Can you work these out from the model? Positions are in its coordinate system, mm. Coordinates: 2 decimals unless noted, no trailing zeros. Write each loop counter-clockwise with the first axis right and the second up, starting at its lowest first coordinate (ties: lowest second). Pieces come first, ordered by that corner, then holes.
```python
from build123d import *

# Parameters (mm, degrees)
SKETCH2_W           = 101.6
SKETCH2_H           = 300
BOSS_EXTRUDE1_DEPTH = 25.4
SKETCH3_R           = 6
CUT_EXTRUDE1_DEPTH  = 25.4
SKETCH4_R           = 16
CUT_EXTRUDE2_DEPTH  = 25.4
SKETCH5_R           = 5.25
CUT_EXTRUDE3_DEPTH  = 25.4


with BuildPart() as part:
    # Sketch2 → Boss-Extrude1 (new body)
    with BuildSketch(Plane(origin=(0, 0, 0), x_dir=(1, 0, 0), z_dir=(0, 1, 0))):
        with Locations((50.8, 150)):
            Rectangle(SKETCH2_W, SKETCH2_H)
    extrude(amount=BOSS_EXTRUDE1_DEPTH)

    # Sketch3 → Cut-Extrude1 (cut)
    with BuildSketch(Plane(origin=(0, 25.4, 0), x_dir=(1, 0, 0), z_dir=(0, 1, 0))):
        with Locations(Location((70.8, 275, 0), (0, 0, 270))):
            Circle(SKETCH3_R)
        with Locations(Location((30.8, 275, 0), (0, 0, 270))):
            Circle(SKETCH3_R)
        with Locations(Location((30.8, 175, 0), (0, 0, 270))):
            Circle(SKETCH3_R)
        with Locations(Location((70.8, 175, 0), (0, 0, 270))):
            Circle(SKETCH3_R)
    extrude(amount=-CUT_EXTRUDE1_DEPTH, mode=Mode.SUBTRACT)

    # Sketch4 → Cut-Extrude2 (cut)
    with BuildSketch(Plane(origin=(0, 25.4, 0), x_dir=(1, 0, 0), z_dir=(0, 1, 0))):
        with Locations(Location((40, 40, 0), (0, 0, 270))):
            Circle(SKETCH4_R)
    extrude(amount=-CUT_EXTRUDE2_DEPTH, mode=Mode.SUBTRACT)

    # Sketch5 → Cut-Extrude3 (cut)
    with BuildSketch(Plane(origin=(0, 25.4, 0), x_dir=(1, 0, 0), z_dir=(0, 1, 0))):
        with Locations(Location((70, 85, 0), (0, 0, 270))):
            Circle(SKETCH5_R)
    extrude(amount=-CUT_EXTRUDE3_DEPTH, mode=Mode.SUBTRACT)


solid = part.part
```
1. If we section it at B-B, the plane z = -175: List the corners of the cut face in (x, y) for me, plus the area to 3 significant figures.
2. If we section it at A-A, the plane z = -40: List the corners of the cut face in (x, y) for me.
3. We'd pull the mould along Z, two halves only. Please class faces 1 (the face through (50, 13, 0)), 2 (the face through (0, 13, -148)), 3 (the face through (27.15, 12.88, -179.76)): released by +Z, released by -Z, zero draft, split by the parting line, or undercut.
4. If I drill on L1, parallel to X at y = 5, z = -175; L2, parallel to X at y = 5.25, z = -40; L3, parallel to Z at x = 29, y = 21, over which ranges is the centre line in solid material (lowest first)?
5. If we section it at D-D, the plane y = 20.25: List the corners of the cut face in (x, z) for me, plus the area to 3 significant figures.
6. If we section it at C-C, the plane x = 30.8: List the corners of the cut face in (y, z) for me, plus the area to 3 significant figures.
Answers:
1. outline: (0, 0) - (24.8, 0) - (24.8, 25.4) - (0, 25.4) - close; (36.8, 0) - (64.8, 0) - (64.8, 25.4) - (36.8, 25.4) - close; (76.8, 0) - (101.6, 0) - (101.6, 25.4) - (76.8, 25.4) - close
1. area: 1,970 mm2
2. outline: (0, 0) - (24, 0) - (24, 25.4) - (0, 25.4) - close; (56, 0) - (101.6, 0) - (101.6, 25.4) - (56, 25.4) - close
3. face 1: released by +Z
3. face 2: zero draft
3. face 3: undercut
4. L1: x = 0 to 24.8, 36.8 to 64.8, 76.8 to 101.6
4. L2: x = 0 to 24, 56 to 101.6
4. L3: z = -300 to -280.72, -269.28 to -180.72, -169.28 to -51.62, -28.38 to 0
5. outline: (0, -300) - (101.6, -300) - (101.6, 0) - (0, 0) - close; hole circle Ø32 at (40, -40); hole circle Ø12 at (30.8, -275); hole circle Ø12 at (30.8, -175); hole circle Ø10.5 at (70, -85); hole circle Ø12 at (70.8, -275); hole circle Ø12 at (70.8, -175)
5. area: 29,100 mm2
6. outline: (0, -300) - (25.4, -300) - (25.4, -281) - (0, -281) - close; (0, -269) - (25.4, -269) - (25.4, -181) - (0, -181) - close; (0, -169) - (25.4, -169) - (25.4, -53.09) - (0, -53.09) - close; (0, -26.91) - (25.4, -26.91) - (25.4, 0) - (0, 0) - close
6. area: 6,350 mm2
